Read the model definition and answer for the solid it produces. Units are mm, in the model's axes. A direction names the side the tool comes from. Round coordinates to 2 decimals unless told otherwise and drop trailing zeros. Order: outer loops, then holes, each group sorted by start corner. A loop starts at its lowest first (then second) coordinate and runs counter-clockwise, first axis right, second up. Notation, with made-up numbers: M 26.5,10 L 55.5,10 A24 ccw 55.5,41 Z; hole C 88,-0.5 d10. An arc over 180 degrees is marked long. Answer as CSV lines item,"result".
```python
from build123d import *

# Parameters (mm, degrees)
SKETCH1_R          = 40
BASE_FLANGE1_DEPTH = 5
CUT_EXTRUDE1_REACH = 58.789
SKETCH6_R          = 2.5
CIRPATTERN1_COUNT  = 16


# Sheet-metal steps are written as plain solids
with BuildPart() as part:
    # Sketch1 → Base-Flange1 (new body)
    with BuildSketch(Plane.XY):
        Circle(SKETCH1_R)
        with BuildLine():
            Line((2.655183609, 1.6), (-2.655183609, 1.6))
            ThreePointArc((-2.655183609, 1.6), (0, -3.1), (2.655183609, 1.6))
        make_face(mode=Mode.SUBTRACT)
    extrude(amount=-BASE_FLANGE1_DEPTH)

    # Sketch6 → Cut-Extrude1 (cut, up to next)
    with BuildSketch(Plane.XY, mode=Mode.PRIVATE) as cut_extrude1_sk1:
        with Locations((0, 30)):
            Circle(SKETCH6_R)
    cut_extrude1_tool1 = extrude(cut_extrude1_sk1.sketch, amount=-CUT_EXTRUDE1_REACH, mode=Mode.PRIVATE) & part.part
    cut_extrude1 = cut_extrude1_tool1.solids().sort_by_distance((0, 30, 0))[0]
    add(cut_extrude1, mode=Mode.SUBTRACT)

    # CirPattern1: Cut-Extrude1 ×16 about axis
    cirpattern1_axis = Axis((0, 0, 0), (0, 0, 1))
    for i in range(1, CIRPATTERN1_COUNT):
        add(cut_extrude1.rotate(cirpattern1_axis, i * 360 / CIRPATTERN1_COUNT), mode=Mode.SUBTRACT)


solid = part.part
```
Item 1: Flat-ended cylindrical pins translate along their axes: pin 1 (1.5 mm diameter, centred on y = 27, z = -3, fed in from -X); pin 2 (4 mm diameter, centred on x = 28.5, y = -10, fed in from +Z); pin 3 (3 mm diameter, centred on y = -3, z = -2.5, fed in from +X); pin 4 (1 mm diameter, centred on y = -27.5, z = -3.5, fed in from +X). Find the tip coordinate at first contact, or state that the pin passes through.
Ans:
pin 1,"x = -30.18"
pin 2,"z = 0"
pin 3,"x = 39.97"
pin 4,"x = 29.51"
Item 2: A cutting plane is placed at A-A, the plane z = -2.3. Give the number of separate pieces and of enclosed holes in the cut face, and give its area (3 significant figures).
Ans:
separate pieces,"1"
enclosed holes,"17"
area,"4,690 mm2"
Item 3: Find the intervals of material crossed by probe 1 along Y at (x, z) = (0, -3.5); probe 2 along X at (y, z) = (20.5, -0.5); probe 3 along Y at (x, z) = (1, -1), in increasing order. Write a range as [from, to].
Ans:
probe 1,"[-40, -32.5], [-27.5, -3.1], [1.6, 27.5], [32.5, 40]"
probe 2,"[-34.35, -23.61], [-18.82, 18.82], [23.61, 34.35]"
probe 3,"[-39.99, -32.29], [-27.71, -2.93], [1.6, 27.71], [32.29, 39.99]"
Item 4: Determine the mould class of faces 1 (the face through (25.7, -10, -2.5)), 2 (the face through (-1, -8, -5)) for opening direction Y: +Y half, -Y half, draft (parallel to the pull), parting line (faces both ways), or undercut.
Ans:
face 1,"undercut"
face 2,"draft"
Item 5: A tool of negligible diameter and unlimited length cuts with its end or side. For faces 3 (the face through (0, 1.6, -2)), 4 (the face through (-1, -8, 0)), from which of +Z, -Z, +X, -X, +Y, -Y can it reach the whole face along a straight path? Write none if from no direction.
Ans:
face 3,"+Z, -Z"
face 4,"+Z, +X, -X, +Y, -Y"
Item 6: A cutting plane is placed at B-B, the plane y = 7.5. Determine the outline of the cut face in (x, z).
Ans:
outline,"M -39.29,-5 L 39.29,-5 L 39.29,0 L -39.29,0 Z"
